Autodesk Inventor part; units mm, degrees
ref_plane "Plano de trabalho1" through (3.2499, 0, 0) normal (0, 0, 1) x (1, 0, 0)
ref_plane "Plano de trabalho2" through (-7.5, 0, 0) normal (0, 0, 1) x (1, 0, 0)
ref_plane "YZ Plane" through (0, 0, 0) normal (1, 0, 0) x (0, 1, 0)
sketch "Esboço1" plane through (0, 0, 0) normal (0, 1, 0) x (-1, 0, 0)
  line L0 (-7.5, 0) -> (-7.5, -11.5)
  line L1 (-7.5, -11.5) -> (7.5, -11.5)
  line L2 (7.5, -11.5) -> (7.5, 0)
  line L3 (-6, -10) -> (-6, 0)
  line L4 (6, 0) -> (6, -10)
  line L5 (6, -10) -> (-6, -10)
  line L6 (7.5, 0) -> (6, 0)
  line L7 (-6, 0) -> (-7.5, 0)
  arc A0 (-3.2499, 0) -> (-3.2501, -10) centre (-0.0795, -5.0001) ccw
  line L8 (-3.2501, -10) -> (3.2501, -10)
  arc A1 (3.2501, -10) -> (3.2499, 0) centre (0.0795, -5.0001) ccw
  line L9 (3.2499, 0) -> (-3.2499, 0)
  line L10 (6, -10) -> (-6, -10)
  line L11 (-6, -10) -> (-6, 0)
  line L12 (-6, 0) -> (6, 0)
  line L13 (6, 0) -> (6, -10)
  point P0 (0, 0)
  point P1 (-3.2499, 0)
  dimension "d0" = 15
  dimension "d1" = 11.5
  dimension "d2" = 1.5
  dimension "d3" = 11.5
extrude "Extrusão1" add sketch "Esboço1" along normal blind 13.5 contours L7 L3 L5 L4 L6 L2 L1 L0 | L12 A0 L3 | A0 L5 L3 | L12 L4 A1 | A1 L4 L5
sketch "Esboço2" plane through (0, 13.5, 0) normal (0, 1, 0) x (1, 0, 0)
  line L0 (-3.2501, 10) -> (3.2501, 10)
  line L1 (7.5, 11.5) -> (-7.5, 11.5)
  line L2 (-3.2501, 10) -> (3.2499, 10)
  line L3 (3.2499, 10) -> (3.2499, 11.5)
  line L4 (3.2499, 11.5) -> (-3.2501, 11.5)
  line L5 (-3.2501, 11.5) -> (-3.2501, 10)
  point P0 (0, 0)
  dimension "d8" = 6.5
extrude "Extrusão2" add sketch "Esboço2" along normal blind 5
sketch "Esboço3" plane through (-3.2501, 0, -10) normal (0, 0, 1) x (1, 0, 0)
  line L0 (0, 13.5) -> (0, 18.5)
  line L1 (6.5, 13.5) -> (6.5, 18.5)
  line L2 (0, 14.8) -> (6.5, 14.8)
  line L3 (6.5, 14.8) -> (6.5, 15.3)
  line L4 (6.5, 15.3) -> (0, 15.3)
  line L5 (0, 15.3) -> (0, 14.8)
  line L6 (6.5, 18.5) -> (0, 18.5)
  line L7 (0, 18.5) -> (6.5, 18.5)
  line L8 (6.5, 18.5) -> (6.5, 18)
  line L9 (6.5, 18) -> (0, 18)
  line L10 (0, 18) -> (0, 18.5)
  line L11 (0, 17.2) -> (6.5, 17.2)
  line L12 (6.5, 17.2) -> (6.5, 16.7)
  line L13 (6.5, 16.7) -> (0, 16.7)
  line L14 (0, 16.7) -> (0, 17.2)
  point P0 (3.2501, 0)
  point P1 (0, 15.3)
  point P2 (6.5, 14.8)
  point P3 (0, 16.7)
  point P4 (6.5, 17.2)
  dimension "d11" = 0.5
  dimension "d12" = 0.5
  dimension "d13" = 0.5
extrude "Extrusão3" add sketch "Esboço3" along normal blind 1 contours L0 L4 L1 L2 | L0 L6 L1 L9
extrude "Extrusão4" add sketch "Esboço3" along normal blind 0.5 contours L0 L11 L1 L13
sketch "Esboço4" plane through (0, 13.5, 0) normal (0, 1, 0) x (1, 0, 0)
  line L0 (-3.2501, 10) -> (-3.2501, 11.5)
  line L1 (-3.2501, 11.5) -> (-7.5, 11.5)
  line L2 (-7.5, 11.5) -> (-7.5, 0)
  line L3 (-7.5, 0) -> (-3.2499, 0)
  arc A0 (-3.2501, 10) -> (-3.2499, 0) centre (-0.0795, 5.0001) ccw
  line L4 (3.2499, 11.5) -> (3.2499, 10)
  line L5 (3.2499, 10) -> (3.2501, 10)
  arc A1 (3.2499, 0) -> (3.2501, 10) centre (0.0795, 5.0001) ccw
  line L6 (3.2499, 0) -> (7.5, 0)
  line L7 (7.5, 0) -> (7.5, 11.5)
  line L8 (7.5, 11.5) -> (3.2499, 11.5)
  line L9 (-3.2501, 9) -> (3.2499, 9)
  line L10 (-3.2501, 11.5) -> (-2.7501, 11.5)
  line L11 (-2.7501, 11.5) -> (-2.7501, 9)
  line L12 (-2.7501, 9) -> (-3.2501, 9)
  line L13 (-3.2501, 9) -> (-3.2501, 11.5)
  line L14 (3.2499, 11.5) -> (2.7499, 11.5)
  line L15 (2.7499, 11.5) -> (2.7499, 9)
  line L16 (2.7499, 9) -> (3.2499, 9)
  line L17 (3.2499, 9) -> (3.2499, 11.5)
  point P0 (0, 0)
  dimension "d20" = 0.5
  dimension "d21" = 0.5
extrude "Extrusão5" cut sketch "Esboço4" against normal blind 3 contours A0 L3 L2 L1 L0 | L8 L7 L6 A1 L4
sketch "Esboço5" plane through (0, 18.5, 0) normal (0, 1, 0) x (1, 0, 0)
  line L0 (-7.5, 11.5) -> (-3.2501, 11.5)
  line L1 (-3.2501, 9) -> (3.2499, 9)
  line L2 (-3.2501, 11.5) -> (-2.7501, 11.5)
  line L3 (-2.7501, 11.5) -> (-2.7501, 9)
  line L4 (-2.7501, 9) -> (-3.2501, 9)
  line L5 (-3.2501, 9) -> (-3.2501, 11.5)
  line L6 (3.2499, 11.5) -> (3.2499, 9)
  line L7 (3.2499, 11.5) -> (2.7499, 11.5)
  line L8 (2.7499, 11.5) -> (2.7499, 9)
  line L9 (2.7499, 9) -> (3.2499, 9)
  line L10 (3.2499, 9) -> (3.2499, 11.5)
  point P0 (0, 0)
  dimension "d22" = 0.5
  dimension "d23" = 0.5
extrude "Extrusão6" cut sketch "Esboço5" against normal up to surface (8 mm away)
sketch "Esboço6" plane through (3.2499, 0, 0) normal (0, 0, 1) x (1, 0, 0)
  point P0 (-3.2499, 0)
ref_plane "Plano de trabalho1" through (3.2499, 0, 0) normal (0, 0, 1) x (1, 0, 0)
sketch "Esboço7" plane through (3.2499, 0, 0) normal (0, 0, 1) x (1, 0, 0)
  line L0 (4.2501, 0) -> (4.2501, 10.5)
  line L1 (4.2501, 10.5) -> (4.2501, 0)
  circle A0 centre (6.9929, 5.2499) radius 1.5
  circle A1 centre (6.9929, 5.2499) radius 2.25
  line L2 (6.9929, 7.4999) -> (4.2501, 7.4999)
  line L3 (6.9929, 2.9999) -> (4.2501, 2.9999)
  line L4 (4.2501, 5.2499) -> (4.7429, 5.2499)
  line L5 (5.4929, 5.2499) -> (9.7501, 5.2499)
  point P0 (-3.2499, 0)
  dimension "d28" = 3
  dimension "d29" = 4.5
extrude "Extrusão7" add sketch "Esboço7" against normal blind 3
ref_plane "Plano de trabalho2" through (-7.5, 0, 0) normal (0, 0, 1) x (1, 0, 0)
sketch "Esboço8" plane through (-7.5, 0, 0) normal (0, 0, 1) x (1, 0, 0)
  circle A0 centre (17.7428, 5.2499) radius 1.5
  line L0 (15, 10.5) -> (10.7499, 10.5)
  line L1 (10.7499, 0) -> (10.7499, 10.5)
  line L2 (10.7499, 0) -> (15, 0)
  line L3 (15, 0) -> (15, 2.9999)
  line L4 (15, 2.9999) -> (17.7428, 2.9999)
  arc A1 (17.7428, 2.9999) -> (17.7428, 7.4999) centre (17.7428, 5.2499) ccw
  line L5 (17.7428, 7.4999) -> (15, 7.4999)
  line L6 (15, 7.4999) -> (15, 10.5)
  circle A2 centre (-2.7428, 5.2499) radius 1.5
  line L7 (0, 0) -> (0, 2.9999)
  line L8 (0, 2.9999) -> (-2.7428, 2.9999)
  arc A3 (-2.7428, 7.4999) -> (-2.7428, 2.9999) centre (-2.7428, 5.2499) ccw
  line L9 (-2.7428, 7.4999) -> (0, 7.4999)
  line L10 (0, 7.4999) -> (0, 10.5)
  line L11 (0, 0) -> (0, 10.5)
  line L12 (0, 10.5) -> (0, 0)
  point P0 (7.5, 0)
extrude "Extrusão8" add sketch "Esboço8" against normal blind 3 contours L8 A3 L9 L11
sketch "Esboço9" plane through (7.5, 0, -11.5) normal (0, 0, -1) x (-1, 0, 0)
  line L0 (10.2501, 18) -> (10.2501, 17.2)
  line L1 (10.2501, 17.2) -> (4.7501, 17.2)
  line L2 (4.7501, 17.2) -> (4.7501, 18)
  line L3 (4.7501, 18) -> (10.2501, 18)
  line L4 (10.2501, 18.5) -> (10.2501, 18)
  line L5 (10.2501, 18) -> (4.7501, 18)
  line L6 (4.7501, 18) -> (4.7501, 18.5)
  line L7 (4.7501, 18.5) -> (10.2501, 18.5)
  point P0 (7.5, 0)
extrude "Extrusão9" cut sketch "Esboço9" against normal blind 10
sketch "Esboço10" plane through (-2.7501, 15.3, -10) normal (0, 0, 1) x (1, 0, 0)
  line L0 (0, 1.4) -> (0, 0)
  line L1 (0, 0) -> (5.5, 0)
  line L2 (5.5, 0) -> (5.5, 1.4)
  line L3 (5.5, 1.4) -> (0, 1.4)
  line L4 (0, 1.9) -> (0, 1.4)
  line L5 (0, 1.4) -> (5.5, 1.4)
  line L6 (5.5, 1.4) -> (5.5, 1.9)
  line L7 (5.5, 1.9) -> (0, 1.9)
  point P0 (2.7501, -15.3)
extrude "Extrusão10" add sketch "Esboço10" along normal up to surface (1 mm away)
fillet "Arredondamento1" radius 2 2 edges at (7.5, 5.25, -11.5) (-7.5, 5.25, -11.5)
properties part number "Suporte Externo - Motor"
Read the model definition and answer for the solid it produces. Units are mm, in the model's axes. A direction names the side the tool comes from. Round coordinates to 2 decimals unless told otherwise and drop trailing zeros. Write each loop counter-clockwise with the first axis right and the second up, starting at its lowest first coordinate (ties: lowest second). Pieces come first, ordered by that corner, then holes.
1. Determine the mould class of faces 1 (the face through (6, 5, -5)), 2 (the face through (6.93, 5.32, -10.9)), 3 (the face through (8.744, 5.316, -1.479)), 4 (the face through (-6, 5, 0)) for opening direction X: pulls with the +X half, pulls with the -X half, needs draft (parallel to the pull), parting line crosses it, or undercut.
2. Which of the six approach directions +Z, -Z, +X, -X, +Y, -Y give full straight-line access (tool end or side, diameter ignored) to faces 5 (the face through (0, 7, -10)), 6 (the face through (9, 3, -1)), 7 (the face through (-9, 3, -1)), 8 (the face through (-9, 7.5, -1)), 9 (the face through (-6, 5, -5))?
3. The part is cut by section D-D, the plane z = -8.5. Determine the outline of the cut face in (x, y), then the cut area to 3 significant figures.
4. The part is cut by section A-A, the plane z = -1.5. Determine the outline of the cut face in (x, y).
5. The part is cut by section B-B, the plane x = -4.5. Determine the outline of the cut face in (y, z), then the cut area to 3 significant figures.
6. The part is cut by section C-C, the plane y = 2.25. Determine the outline of the cut face in (x, z), then the cut area to 3 significant figures.
7. Given pin 1 Ø5 at (x, y) = (4, 8.5) entering from +Z; pin 2 Ø3 at (x, z) = (9.5, -1.5) entering from +Y; pin 3 Ø3 at (y, z) = (9.5, -4.5) entering from +X; pin 4 Ø1.3 at (x, y) = (-9.5, 4.5) entering from -Z, each flat-ended and moving along its own axis, determine where each tip first touches the part or whether it passes through.
8. Straight lines are drawn through the part: L1, parallel to Y at x = -6.25, z = -7.5; L2, parallel to Z at x = 4.25, y = 1.25; L3, parallel to X at y = 9, z = -2.75. For each, find the intervals that lie inside material, in ascending order.
Values:
1. face 1: undercut
1. face 2: pulls with the +X half
1. face 3: undercut
1. face 4: needs draft
2. face 5: +Z, -Y
2. face 6: +Z, -Z, +X, -Y
2. face 7: +Z, -Z, -X, -Y
2. face 8: +Z, -Z, -X, +Y
2. face 9: +Y, -Y
3. outline: (-7.5, 0) - (-4.85, 0) - (-4.85, 10.5) - (-7.5, 10.5) - close; (4.85, 0) - (7.5, 0) - (7.5, 10.5) - (4.85, 10.5) - close
3. area: 55.6 mm2
4. outline: (-10.24, 3) - (-7.5, 3) - (-7.5, 0) - (-4.85, 0) - (-4.85, 10.5) - (-7.5, 10.5) - (-7.5, 7.5) - (-10.24, 7.5) arc R2.25 ccw to start; (4.85, 0) - (7.5, 0) - (7.5, 3) - (10.24, 3) arc R2.25 ccw to (10.24, 7.5) - (7.5, 7.5) - (7.5, 10.5) - (4.85, 10.5) - close; hole circle Ø3 at (-10.24, 5.25); hole circle Ø3 at (10.24, 5.25)
5. outline: (0, -11.5) - (10.5, -11.5) - (10.5, -8.94) - (0, -8.94) - close; (0, -1.06) - (10.5, -1.06) - (10.5, 0) - (0, 0) - close
5. area: 38.0 mm2
6. outline: (-7.5, -9.5) arc R2 ccw to (-5.5, -11.5) - (5.5, -11.5) arc R2 ccw to (7.5, -9.5) - (7.5, 0) - (3.25, 0) arc R5.92 cw to (3.25, -10) - (-3.25, -10) arc R5.92 cw to (-3.25, 0) - (-7.5, 0) - close
6. area: 67.0 mm2
7. pin 1: stops at z = 0
7. pin 2: stops at y = 7.5
7. pin 3: stops at x = 7.5
7. pin 4: stops at z = -3
8. L1: y = 0 to 10.5
8. L2: z = -11.5 to -9.2, -0.8 to 0
8. L3: x = -7.5 to -5.56, 5.56 to 7.5
